Work out the finished part from the listing and answer in its coordinate system (mm). A direction names the side the tool comes from. Round coordinates to 2 decimals unless told otherwise and drop trailing zeros. Write each loop counter-clockwise with the first axis right and the second up, starting at its lowest first coordinate (ties: lowest second). Pieces come first, ordered by that corner, then holes. Notation, with made-up numbers: (42.5, 84.5) - (74.5, 84.5) arc R24 cw to (74.5, 107.5) - close; hole circle Ø6 at (20.5, 82). An arc over 180 degrees is marked (long way). Answer as a JSON object with one key per item and string values.
Autodesk Inventor part; units mm, degrees
ref_plane "YZ Plane" through (0, 0, 0) normal (1, 0, 0) x (0, 1, 0)
ref_plane "XZ Plane" through (0, 0, 0) normal (0, 1, 0) x (-1, 0, 0)
ref_plane "XY Plane" through (0, 0, 0) normal (0, 0, 1) x (1, 0, 0)
sketch "Sketch1" plane through (0, 0, 0) normal (0, 0, 1) x (1, 0, 0)
  circle A0 centre (0, 0) radius 3.5
  dimension "d0" = 7
extrude "Extrusion1" add sketch "Sketch1" along normal blind 3
sketch "Sketch4" plane through (0, 0, 0) normal (0, 0, 1) x (1, 0, 0)
  circle A0 centre (0, 0) radius 3.5
  line L0 (2.0207, 3.5) -> (4.0415, 0)
  line L1 (4.0415, 0) -> (2.0207, -3.5)
  line L2 (2.0207, -3.5) -> (-2.0207, -3.5)
  line L3 (-2.0207, -3.5) -> (-4.0415, 0)
  line L4 (-4.0415, 0) -> (-2.0207, 3.5)
  line L5 (-2.0207, 3.5) -> (2.0207, 3.5)
  point P0 (0, 3.5)
extrude "Extrusion4" add sketch "Sketch4" against normal blind 1.5
fillet "Fillet1" radius 1 1 edges at (-3.5, 0, 3)
sketch "Sketch5" plane through (0, 0, 3) normal (0, 0, 1) x (1, 0, 0)
  circle A0 centre (0, 0) radius 2.5
  dimension "d14" = 5
extrude "Extrusion5" cut sketch "Sketch5" against normal blind 0.5
sketch "Sketch6" plane through (0, 0, 0) normal (0, 0, 1) x (1, 0, 0)
  circle A0 centre (0, 0) radius 2.5
  circle A1 centre (0, 0) radius 2
  dimension "d17" = 4
extrude "Extrusion6" cut sketch "Sketch6" along normal mid plane 16 contours A1
properties part number "bolt"
Item 1: Consider line 1 along Y through (x, z) = (0, 0.4); line 2 along X through (y, z) = (1, -0.75). Determine where each line is inside the solid, lowest interval first.
Results found:
{"line 1": "-3.5 to -2, 2 to 3.5", "line 2": "-3.46 to -1.73, 1.73 to 3.46"}
Item 2: For faces 1 (the flat face through (1.85, 3.15, 0)), 2 (the flat face through (3.65, 0.01, 0)), 3 (the flat face through (-1.86, 3.15, 0)), 4 (the flat face through (-1.9, -3.2, 0)), 5 (the cylindrical face through (3.233, 1.341, 0.986)), determine the directions among +Z, -Z, +X, -X, +Y, -Y from which every point of the face is accessible in a straight line to the end or side of a thin tool.
Results found:
{"face 1": "+Z, +X, +Y", "face 2": "+Z, +X", "face 3": "+Z, -X, +Y", "face 4": "+Z, -X, -Y", "face 5": "+Z"}
Item 3: A cutting plane is placed at B-B (z = 1). Write down the section's boundary in (x, y), and give its area (3 significant figures).
Results found:
{"outline": "circle Ø7 at (0, 0); hole circle Ø4 at (0, 0)", "area": "25.9 mm²"}
Item 4: A cutting plane is placed at A-A (z = -0.75). Write down the section's boundary in (x, y), and give its area (3 significant figures).
Results found:
{"outline": "(-4.04, 0) - (-2.02, -3.5) - (2.02, -3.5) - (4.04, 0) - (2.02, 3.5) - (-2.02, 3.5) - close; hole circle Ø4 at (0, 0)", "area": "29.9 mm²"}
Item 5: Determine the mould class of faces 6 (the cylindrical face through (0, -2, 1)), 7 (the flat face through (-3, -1.8, -0.7)), 8 (the flat face through (3, 1.8, -0.7)), 9 (the flat face through (-3.7, 0, 0)) for opening direction X: pulls with the +X half, pulls with the -X half, needs draft (parallel to the pull), parting line crosses it, or undercut.
Results found:
{"face 6": "undercut", "face 7": "pulls with the -X half", "face 8": "pulls with the +X half", "face 9": "needs draft"}
Item 6: Each of these flat-tipped pins is pushed along its axis until it touches: P1, Ø0.5, axis at x = -1, y = -2.5, coming from the +Z side; P2, Ø0.5, axis at x = 1, y = 3, coming from the +Z side; P3, Ø0.5, axis at x = 3.5, y = 0.5, coming from the +Z side; P4, Ø3.5, axis at x = 0, y = 0, coming from the -Z side. Where does it stop, or does it pass through?
Results found:
{"P1": "z = 3", "P2": "z = 2.91", "P3": "z = 2.62", "P4": "through"}
